Part model, mm, in its own coordinate system. Face numbers are marked on the shaded views. A direction names the side the tool comes from. Give positions to 0.01 mm unless a question says otherwise; leave off trailing zeros. Write each loop counter-clockwise with the first axis right and the second up, starting at its lowest first coordinate (ties: lowest second). Pieces come first, ordered by that corner, then holes. Notation, with made-up numbers: M 67.5,32.5 L 87.5,32.5 A22 cw 87.5,50.5 Z; hole C 22,-5.75 d8. An arc over 180 degrees is marked long. Answer as CSV lines item,"result". Start each with the question number.
1) Slice it at D-D, the plane y = -11.5. Give the cut face in (x, z).
2) Mould opens along Y. For the marked faces 3, 4 and 5 say: pulls with the +Y half, pulls with the -Y half, needs draft (parallel to the pull), parting line crosses it, or undercut.
3) Pin check, flat tips, straight feed: pin 1 Ø7.5 at (y, z) = (-9, -20) entering from -X; pin 2 Ø2.5 at (y, z) = (-9, -14) entering from +X; pin 3 Ø17 at (x, y) = (3.5, 0) entering from +Z. Stop position of each tip, or through.
4) Slice it at B-B, the plane y = 0. Give the cut face in (x, z), plus the area to 3 significant figures.
5) Wall check: line 1 along X through (y, z) = (0, 11); line 2 along Y through (x, z) = (3.5, 11.5); line 3 along Z through (x, y) = (22.5, -12.5). Give the ranges that are in metal, low to high. Write a range as from..to.
6) Tool access for the marked faces 1 and 2: list every direction of +Z, -Z, +X, -X, +Y, -Y with a clear straight run to the whole face (end or side of a thin tool).
7) Slice it at C-C, the plane z = 1. Give the cut face in (x, y), plus the area to 3 significant figures.
8) Slice it at A-A, the plane x = 3.5. Give the cut face in (y, z).
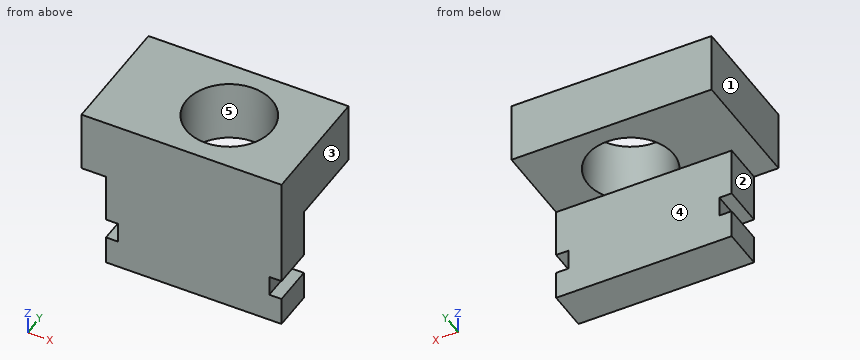
```python
from build123d import *

# Parameters (mm, degrees)
SKETCH1_W           = 49
SKETCH1_H           = 30
BOSS_EXTRUDE1_DEPTH = 15
SKETCH3_R           = 10.5
CUT_EXTRUDE1_DEPTH  = 23
SKETCH4_W           = 43
SKETCH4_H           = 10
BOSS_EXTRUDE3_DEPTH = 24
SKETCH5_W           = 5
SKETCH5_H           = 10
CUT_EXTRUDE2_DEPTH  = 3


with BuildPart() as part:
    # Sketch1 → Boss-Extrude1 (new body)
    with BuildSketch(Plane.XY):
        Rectangle(SKETCH1_W, SKETCH1_H)
    extrude(amount=BOSS_EXTRUDE1_DEPTH)

    # Sketch3 → Cut-Extrude1 (cut)
    with BuildSketch(Plane(origin=(0, 0, 0), x_dir=(-1, 0, 0), z_dir=(0, 0, -1))):
        with Locations((-3.5, 0)):
            Circle(SKETCH3_R)
    extrude(amount=-CUT_EXTRUDE1_DEPTH, mode=Mode.SUBTRACT)

    # Sketch4 → Boss-Extrude3 (add)
    with BuildSketch(Plane(origin=(0, 0, 0), x_dir=(-1, 0, 0), z_dir=(0, 0, -1))):
        with Locations((-3, -10)):
            Rectangle(SKETCH4_W, SKETCH4_H)
    extrude(amount=BOSS_EXTRUDE3_DEPTH)

    # Sketch5 → Cut-Extrude2 (cut)
    with BuildSketch(Plane.ZY.offset(18.5)):
        with Locations((-14.5, -10)):
            Rectangle(SKETCH5_W, SKETCH5_H)
    cut_extrude2 = extrude(amount=-CUT_EXTRUDE2_DEPTH, mode=Mode.SUBTRACT)

    # Mirror1: Cut-Extrude2 across plane
    add(cut_extrude2.mirror(Plane.ZY.offset(-3)), mode=Mode.SUBTRACT)


solid = part.part
```
Found:
1,outline,"M -24.5,0 L -18.5,0 L -18.5,-12 L -15.5,-12 L -15.5,-17 L -18.5,-17 L -18.5,-24 L 24.5,-24 L 24.5,-17 L 21.5,-17 L 21.5,-12 L 24.5,-12 L 24.5,15 L -24.5,15 Z"
2,face 3,"needs draft"
2,face 4,"pulls with the +Y half"
2,face 5,"undercut"
3,pin 1,"x = -18.5"
3,pin 2,"x = 21.5"
3,pin 3,"z = 0"
4,outline,"M -24.5,0 L -7,0 L -7,15 L -24.5,15 Z; M 14,0 L 24.5,0 L 24.5,15 L 14,15 Z"
4,area,"420 mm²"
5,line 1,"-24.5..-7, 14..24.5"
5,line 2,"-15..-10.5, 10.5..15"
5,line 3,"-24..-17, -12..15"
6,face 1,"+Z, -Z, -X, +Y, -Y"
6,face 2,"-Z, -X, +Y, -Y"
7,outline,"M -24.5,-15 L 24.5,-15 L 24.5,15 L -24.5,15 Z; hole C 3.5,0 d21"
7,area,"1,120 mm²"
8,outline,"M -15,-24 L -5,-24 L -5,0 L -10.5,0 L -10.5,15 L -15,15 Z; M 10.5,0 L 15,0 L 15,15 L 10.5,15 Z"
